from build123d import *

# Parameters (mm, degrees)
HOLE_WIZARD_M31_D           = 3.4
HOLE_WIZARD_M31_CBORE_D     = 6.5
HOLE_WIZARD_M31_CBORE_DEPTH = 3


with BuildPart() as part:
    # Эскиз2 → Повернуть1 (revolve)
    with BuildSketch(Plane(origin=(0, 0, 0), x_dir=(0, 0, -1), z_dir=(1, 0, 0)), mode=Mode.PRIVATE) as revolve_1_sk:
        Polygon((0, 0), (0, 16.5), (5, 16.5), (5, 6.3), (49, 6.3), (49, 0), align=None)
    revolve(revolve_1_sk.sketch.rotate(Axis((0, 0, -49), (0, 0, 1)), 90), axis=Axis((0, 0, -49), (0, 0, 1)))

    # Цековка для винта с внутренним шестигранником M31 (through all)
    with Locations(Plane.XY):
        with Locations((-12.5, 0), (0, 12.5), (12.5, 0), (0, -12.5)):
            CounterBoreHole(HOLE_WIZARD_M31_D / 2, HOLE_WIZARD_M31_CBORE_D / 2, HOLE_WIZARD_M31_CBORE_DEPTH)


solid = part.part
The model under review builds one solid part; all positions refer to its coordinate system, in mm. A direction names the side the tool comes from. Coordinates: 2 decimals unless noted, no trailing zeros. Order: outer loops, then holes, each group sorted by start corner. A loop starts at its lowest first (then second) coordinate and runs counter-clockwise, first axis right, second up. Notation, with made-up numbers: (28.25, 29.25) -> (67.25, 29.25) arc R15 ccw to (67.25, 44.25) -> close; hole circle Ø9 at (-30.5, 73.25). An arc over 180 degrees is marked (long way). Answer in a Markdown table with one row per item.
(1) The part is to be moulded in two halves that separate along Y. For faces 4 (the flat face through (0, 7, -5)), 5 (the cylindrical face through (10.93, -0.65, -4.01)), 6 (the cylindrical face through (-15.738, -4.956, -2.535)), say which applies: +Y half, -Y half, draft (parallel to the pull), parting line (faces both ways), or undercut.
Answers:
| item | result |
|---|---|
| face 4 | draft |
| face 5 | undercut |
| face 6 | parting line |
(2) Insertion check: pin 1 (7.5 mm diameter, centred on x = 0, y = -12.5, fed in from -Z); pin 2 (4 mm diameter, centred on x = 0, y = -12.5, fed in from +Z); pin 3 (1.5 mm diameter, centred on y = 4, z = -32, fed in from +X); pin 4 (2 mm diameter, centred on x = -9, z = -21, fed in from -Y). Each pin has a flat end and moves straight along its axis. Give the tip position at first contact, or say it passes through.
Answers:
| item | result |
|---|---|
| pin 1 | z = -5 |
| pin 2 | z = -3 |
| pin 3 | x = 5.4 |
| pin 4 | through |
(3) Machinability: for faces 1 (the cylindrical face through (5, 3.83, -27.31)), 2 (the flat face through (13.9, -1.4, -3)), 3 (the cylindrical face through (0.221, 14.186, -4.014)), which of the approach directions +Z, -Z, +X, -X, +Y, -Y give a long, thin tool a straight path to every point of the face, cutting with its end or side? Answer none if there is none.
Answers:
| item | result |
|---|---|
| face 1 | -Z |
| face 2 | +Z |
| face 3 | +Z, -Z |
(4) Consider section D-D (x = -11.5). Write out the cut boundary in (y, z), plus the area to 3 significant figures.
Answers:
| item | result |
|---|---|
| outline | (-11.83, -5) -> (-1.37, -5) -> (-1.37, -3) -> (-3.09, -3) -> (-3.09, 0) -> (-11.83, 0) -> close; (1.37, -5) -> (11.83, -5) -> (11.83, 0) -> (3.09, 0) -> (3.09, -3) -> (1.37, -3) -> close |
| area | 94.3 mm² |
(5) Consider section A-A (y = 0). Write out the cut boundary in (x, z), plus the area to 3 significant figures.
Answers:
| item | result |
|---|---|
| outline | (-16.5, -5) -> (-14.2, -5) -> (-14.2, -3) -> (-15.75, -3) -> (-15.75, 0) -> (-16.5, 0) -> close; (-10.8, -5) -> (-6.3, -5) -> (-6.3, -49) -> (6.3, -49) -> (6.3, -5) -> (10.8, -5) -> (10.8, -3) -> (9.25, -3) -> (9.25, 0) -> (-9.25, 0) -> (-9.25, -3) -> (-10.8, -3) -> close; (14.2, -5) -> (16.5, -5) -> (16.5, 0) -> (15.75, 0) -> (15.75, -3) -> (14.2, -3) -> close |
| area | 667 mm² |
(6) Wall thickness on line 1 along Y through (x, z) = (0, -3.95); line 2 along Y through (x, z) = (0, -1.9); line 3 along Z through (x, y) = (9, -5): over which ranges is each line inside the solid? List them lowest first.
Answers:
| item | result |
|---|---|
| line 1 | -16.5 to -14.2, -10.8 to 10.8, 14.2 to 16.5 |
| line 2 | -16.5 to -15.75, -9.25 to 9.25, 15.75 to 16.5 |
| line 3 | -5 to 0 |
(7) Consider section C-C (z = -4). Write out the cut boundary in (x, y).
Answers:
| item | result |
|---|---|
| outline | circle Ø33 at (0, 0); hole circle Ø3.4 at (-12.5, 0); hole circle Ø3.4 at (0, -12.5); hole circle Ø3.4 at (0, 12.5); hole circle Ø3.4 at (12.5, 0) |
